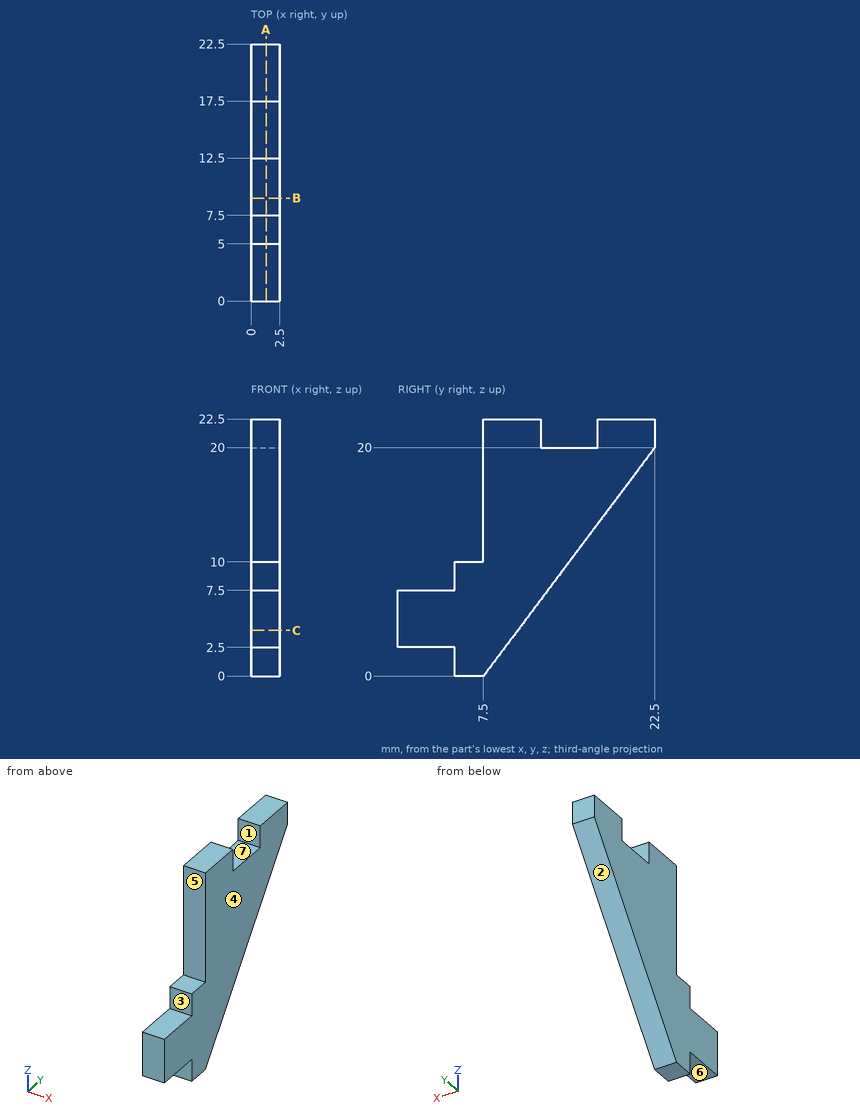
Geometry check sheet. Reference: drawing and pictorial views, mm from the part's lowest x, y, z. A direction names the side the tool comes from. Round coordinates to 2 decimals unless told otherwise and drop trailing zeros. Loops run counter-clockwise (first coordinate to the right, second up) from the corner with the lowest first, then second, coordinate; pieces in that order, holes last. Notation, with made-up numbers: (13.5, 84.25) - (26.5, 84.25) arc R18 ccw to (26.5, 93.25) - close; hole circle Ø1 at (39.5, 19.25). An arc over 180 degrees is marked (long way). Answer in a Markdown table with one row per item. Add a question column.
Q1. Section check A-A on x = 1.3. Enter the section's corners in (y, z), plus the area to 3 significant figures.
Q2. Release check for a two-part mould opening along Y. For the marked faces 1, 2, 3 and 4 record: pulls with the +Y half, pulls with the -Y half, needs draft (parallel to the pull), parting line crosses it, or undercut.
Q3. Tool access check on the marked faces 5, 6 and 7. Record the directions out of +Z, -Z, +X, -X, +Y, -Y that give a thin tool (end or side, any length) a straight path to the whole face; none if there is none.
Q4. Gauge pin test, flat ends, axial feed: pin 1 (1.2 mm diameter, centred on x = 1, y = 2, fed in from -Z); pin 2 (0.8 mm diameter, centred on x = 1, y = 15.5, fed in from +Z); pin 3 (0.8 mm diameter, centred on x = 1.5, z = 21.5, fed in from -Y); pin 4 (4 mm diameter, centred on y = 15.5, z = 7, fed in from -X). Record the tip position at first contact, or that the pin passes through.
Q5. Section check B-B on y = 9. Enter the section's corners in (x, z).
Q6. Section check C-C on z = 4. Enter the section's corners in (x, y), plus the area to 4 significant figures.
Q7. Material ranges on line 1 (Z direction, x = 2.1, y = 6.75); line 2 (Z direction, x = 0.55, y = 3.5); line 3 (Y direction, x = 1.95, z = 13.75), recorded low to high.
Found:
| question | item | result |
|---|---|---|
| 1 | outline | (0, 2.5) - (5, 2.5) - (5, 0) - (7.5, 0) - (22.5, 20) - (22.5, 22.5) - (17.5, 22.5) - (17.5, 20) - (12.5, 20) - (12.5, 22.5) - (7.5, 22.5) - (7.5, 10) - (5, 10) - (5, 7.5) - (0, 7.5) - close |
| 1 | area | 225 mm² |
| 2 | face 1 | undercut |
| 2 | face 2 | pulls with the +Y half |
| 2 | face 3 | pulls with the -Y half |
| 2 | face 4 | needs draft |
| 3 | face 5 | +Z, +X, -X, -Y |
| 3 | face 6 | -Z, +X, -X, -Y |
| 3 | face 7 | +Z, +X, -X |
| 4 | pin 1 | stops at z = 2.5 |
| 4 | pin 2 | stops at z = 20 |
| 4 | pin 3 | stops at y = 7.5 |
| 4 | pin 4 | passes through |
| 5 | outline | (0, 2) - (2.5, 2) - (2.5, 22.5) - (0, 22.5) - close |
| 6 | outline | (0, 0) - (2.5, 0) - (2.5, 10.5) - (0, 10.5) - close |
| 6 | area | 26.25 mm² |
| 7 | line 1 | z = 0 to 10 |
| 7 | line 2 | z = 2.5 to 7.5 |
| 7 | line 3 | y = 7.5 to 17.81 |
